Read the model definition and answer for the solid it produces. Units are mm, in the model's axes. Face numbers are marked on the shaded views. A direction names the side the tool comes from. Give positions to 0.01 mm unless a question says otherwise; leave off trailing zeros. Order: outer loops, then holes, each group sorted by start corner. A loop starts at its lowest first (then second) coordinate and runs counter-clockwise, first axis right, second up. Notation, with made-up numbers: (63, 54) -> (115, 54) arc R26 cw to (115, 86) -> close; hole circle Ø1 at (-23.5, 40). An arc over 180 degrees is marked (long way). Use one line per item in the form item = value.
```python
from build123d import *

# Parameters (mm, degrees)
SKETCH1_R               = 12.5
BOSS_EXTRUDE1_DEPTH     = 40
SKETCH2_W               = 8
SKETCH2_H               = 35
CUT_EXTRUDE1_DEPTH      = 4
SKETCH3_R               = 15.875
BOSS_EXTRUDE2_DEPTH     = 40
SKETCH5_R               = 9.5504
CUT_EXTRUDE2_DEPTH      = 25.4
CUT_EXTRUDE3_REACH      = 85.091
CUT_EXTRUDE3_END_RADIUS = 15.875
SKETCH6_R               = 2.665
CIRPATTERN1_COUNT       = 2
CIRPATTERN1_ANGLE       = 90


with BuildPart() as part:
    # Sketch1 → Boss-Extrude1 (new body)
    with BuildSketch(Plane.XY):
        Circle(SKETCH1_R)
    extrude(amount=BOSS_EXTRUDE1_DEPTH)

    # Sketch2 → Cut-Extrude1 (cut)
    with BuildSketch(Plane(origin=(0, 12.5, 0), x_dir=(1, 0, 0), z_dir=(0, 1, 0))):
        with Locations((0, -20)):
            Rectangle(SKETCH2_W, SKETCH2_H)
    extrude(amount=-CUT_EXTRUDE1_DEPTH, mode=Mode.SUBTRACT)

    # Sketch3 → Boss-Extrude2 (add)
    with BuildSketch(Plane.XY.offset(40)):
        Circle(SKETCH3_R)
    extrude(amount=BOSS_EXTRUDE2_DEPTH)

    # Sketch5 → Cut-Extrude2 (cut)
    with BuildSketch(Plane.XY.offset(80)):
        Circle(SKETCH5_R)
    extrude(amount=-CUT_EXTRUDE2_DEPTH, mode=Mode.SUBTRACT)

    # Cut-Extrude3: up to this cylinder (the profile starts inside it)
    cut_extrude3_end = Plane(origin=(0, 0, 67.3), z_dir=(0, 0, -1)) * Cylinder(CUT_EXTRUDE3_END_RADIUS, 202.932, mode=Mode.PRIVATE)
    # Sketch6 → Cut-Extrude3 (cut, up to the surface)
    with BuildSketch(Plane(origin=(0, 0, 0), x_dir=(1, 0, 0), z_dir=(0, 1, 0)), mode=Mode.PRIVATE) as cut_extrude3_sk1:
        with Locations(Location((0, -67.3, 0), (0, 0, 90))):
            Circle(SKETCH6_R)
    cut_extrude3_tool1 = extrude(cut_extrude3_sk1.sketch, amount=CUT_EXTRUDE3_REACH, mode=Mode.PRIVATE) & cut_extrude3_end
    cut_extrude3 = cut_extrude3_tool1.solids().sort_by_distance((0, 0, 67.3))[0]
    add(cut_extrude3, mode=Mode.SUBTRACT)

    # CirPattern1: Cut-Extrude3 ×2 about axis
    cirpattern1_axis = Axis((0, 0, 80), (0, 0, -1))
    for i in range(1, CIRPATTERN1_COUNT):
        add(cut_extrude3.rotate(cirpattern1_axis, i * CIRPATTERN1_ANGLE / (CIRPATTERN1_COUNT - 1)), mode=Mode.SUBTRACT)


solid = part.part
```
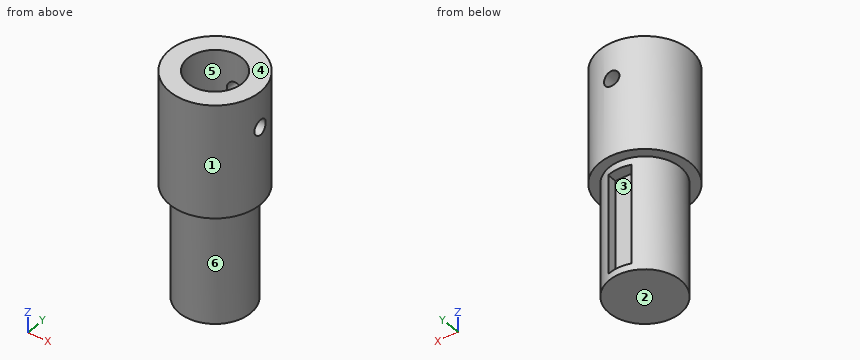
Item 1: The part is cut by section A-A on y = 0. Give the vertices of the cut face in (x, z) (3 decimals), and give its area (3 significant figures).
Checks:
outline = (-15.875, 40) -> (-12.5, 40) -> (-12.5, 0) -> (12.5, 0) -> (12.5, 40) -> (15.875, 40) -> (15.875, 64.635) -> (9.55, 64.635) -> (9.55, 54.6) -> (-9.55, 54.6) -> (-9.55, 80) -> (-15.875, 80) -> close; (9.55, 69.965) -> (15.875, 69.965) -> (15.875, 80) -> (9.55, 80) -> close
area = 1,750 mm²
Item 2: Determine the mould class of the marked faces 1, 2 and 3 for opening direction X: +X half, -X half, draft (parallel to the pull), parting line (faces both ways), or undercut.
Checks:
face_1 = parting line
face_2 = draft
face_3 = undercut
Item 3: The part is cut by section C-C on z = 67.3. Give the vertices of the cut face in (x, y) (3 decimals).
Checks:
outline = (-2.665, 9.171) -> (-2.665, 15.65) arc R15.875 ccw (long way) to (15.65, -2.665) -> (9.171, -2.665) arc R9.55 cw (long way) to start; (2.665, 9.171) arc R9.55 cw to (9.171, 2.665) -> (15.65, 2.665) arc R15.875 ccw to (2.665, 15.65) -> close
Item 4: Straight lines are drawn through the part: L1, parallel to X at y = 8.5, z = 72.5; L2, parallel to Y at x = -5.5, z = 55; L3, parallel to Z at x = 5, y = 6. For each, find the intervals that lie inside material, in ascending order. Write a range as from..to.
Checks:
L1 = -13.41..-4.35, 4.35..13.41
L2 = -14.89..-7.81, 7.81..14.89
L3 = 0..54.6
Item 5: The part is cut by section D-D on x = 11. Give the vertices of the cut face in (y, z) (3 decimals), and give its area (3 significant figures).
Checks:
outline = (-11.446, 40) -> (-5.937, 40) -> (-5.937, 0) -> (5.937, 0) -> (5.937, 40) -> (11.446, 40) -> (11.446, 80) -> (-11.446, 80) -> close; hole circle Ø5.33 at (0, 67.3)
area = 1,370 mm²
Item 6: The part is cut by section B-B on x = 0. Give the vertices of the cut face in (y, z) (3 decimals), and give its area (3 significant figures).
Checks:
outline = (-15.875, 40) -> (-12.5, 40) -> (-12.5, 0) -> (12.5, 0) -> (12.5, 2.5) -> (8.5, 2.5) -> (8.5, 37.5) -> (12.5, 37.5) -> (12.5, 40) -> (15.875, 40) -> (15.875, 64.635) -> (9.55, 64.635) -> (9.55, 54.6) -> (-9.55, 54.6) -> (-9.55, 80) -> (-15.875, 80) -> close; (9.55, 69.965) -> (15.875, 69.965) -> (15.875, 80) -> (9.55, 80) -> close
area = 1,610 mm²
Item 7: Given pin 1 Ø1.5 at (x, y) = (-1.5, -0.5) entering from +Z; pin 2 Ø1.5 at (x, y) = (-11.5, -10.5) entering from -Z; pin 3 Ø8 at (y, z) = (11.5, 58.5) entering from +X, each flat-ended and moving along its own axis, determine where each tip first touches the part or whether it passes through.
Checks:
pin_1 = 54.6
pin_2 = 40
pin_3 = 13.99
Item 8: Which of the six approach directions +Z, -Z, +X, -X, +Y, -Y give full straight-line access (tool end or side, diameter ignored) to the marked faces 4, 5 and 6?
Checks:
face_4 = +Z, +X, -X, +Y, -Y
face_5 = +Z
face_6 = -Z
